The model under review builds one solid part; all positions refer to its coordinate system, in mm. A direction names the side the tool comes from. Coordinates: 2 decimals unless noted, no trailing zeros. Order: outer loops, then holes, each group sorted by start corner. A loop starts at its lowest first (then second) coordinate and runs counter-clockwise, first axis right, second up. Notation, with made-up numbers: (57, 57.25) -> (76, 57.25) arc R17 ccw to (76, 77.25) -> close; hole circle Ø5 at (19, -2.5). An arc over 180 degrees is marked (long way). Use one line per item in the form item = value. Start each with the question number.
(1) Take a section at C-C (y = 10.5). State the section outline as (x, z) points, then the cut area to 3 significant figures.
(2) For faces 1 (the flat face through (56, 0, 15)), 2 (the flat face through (35, 2, 2)), 3 (the flat face through (33.55, -2.5, 6.6)), 4 (the flat face through (36.45, -2.5, 6.6)), 5 (the flat face through (46, 0, 5)), list the 3-axis set-ups (+Z, -Z, +X, -X, +Y, -Y) from which the entire face can be reached by the end or side of a thin tool; tool diameter is ignored.
(3) Take a section at B-B (x = 57.5). State the section outline as (y, z) points, then the cut area to 3 significant figures.
(4) Take a section at D-D (x = 35). State the section outline as (y, z) points, then the cut area to 3 significant figures.
(5) Take a section at A-A (z = 12). State the section outline as (x, y) points.
(6) Wall thickness on line 1 along Z through (x, y) = (57.5, 10.7); line 2 along Z through (x, y) = (35, 3.5); line 3 along Z through (x, y) = (57.5, -1.5): over which ranges is each line inside the solid? List them lowest first.
(7) Mouldability with a two-part tool opening along X and no side actions: class faces 6 (the flat face through (33.55, -2.5, 17.3)), 7 (the cylindrical face through (36.6, 1.56, 11.93)), 8 (the flat face through (32, -2, 12)), 9 (the flat face through (36.45, -2.5, 17.3)) as +X half, -X half, draft (parallel to the pull), parting line (faces both ways), or undercut.
(8) Insertion check: pin 1 Ø12 at (x, y) = (56, 1.5) entering from +Z; pin 2 Ø0.5 at (y, z) = (-2.5, 19) entering from -X; pin 3 Ø1.5 at (y, z) = (-5.5, 16.5) entering from -X. Each pin has a flat end and moves straight along its axis. Give the tip position at first contact, or say it passes through.
```python
from build123d import *

# Parameters (mm, degrees)
MAIN_DEPTH                   = 22
ESQUISSE2_W                  = 10
ESQUISSE2_H                  = 8
ENL_V_MAT_EXTRU_1_DEPTH      = 19
ESQUISSE3_W                  = 21
ESQUISSE3_H                  = 10
ENL_V_MAT_EXTRU_2_DEPTH      = 10
ESQUISSE4_R                  = 3
ENL_V_MAT_EXTRU_3_DEPTH      = 1
ENL_V_MAT_EXTRU_3_DEPTH_BACK = 25
CONG_2_R                     = 5
ENL_V_START                  = -18
ESQUISSE6_W                  = 7
ESQUISSE6_H                  = 24
ENL_V_MAT_EXTRU_4_DEPTH      = 18
SKETCH1_W                    = 10
SKETCH1_H                    = 2
CUT_EXTRUDE1_DEPTH           = 19
SKETCH2_R                    = 1.6
CUT_EXTRUDE2_DEPTH           = 19
FILLET1_R                    = 1.5
CONG_3_R                     = 3
SKETCH3_W                    = 22
SKETCH3_H                    = 24
CUT_EXTRUDE3_DEPTH           = 39


with BuildPart() as part:
    # Esquisse1 → Main (new body)
    with BuildSketch(Plane.XY):
        Polygon((-12, -12), (12, -12), (12, -2), (15.55, -2), (15.55, -3), (18.45, -3), (18.45, -2), (22, -2), (22, 6), (12, 6), (12, 12), (-12, 12), align=None)
    extrude(amount=MAIN_DEPTH)

    # Esquisse2 → Enlèv. mat.-Extru.1 (cut, through all)
    with BuildSketch(Plane(origin=(6, 0, 0), x_dir=(0, 0, -1), z_dir=(1, 0, 0))):
        with Locations((-5, 2)):
            Rectangle(ESQUISSE2_W, ESQUISSE2_H)
    extrude(amount=-ENL_V_MAT_EXTRU_1_DEPTH, mode=Mode.SUBTRACT)

    # Esquisse3 → Enlèv. mat.-Extru.2 (cut)
    with BuildSketch(Plane(origin=(0, 0, 0), x_dir=(-1, 0, 0), z_dir=(0, 0, -1))):
        with Locations((1.5, -7)):
            Rectangle(ESQUISSE3_W, ESQUISSE3_H)
    extrude(amount=-ENL_V_MAT_EXTRU_2_DEPTH, mode=Mode.SUBTRACT)

    # Esquisse4 → Enlèv. mat.-Extru.3 (cut, two sides)
    with BuildSketch(Plane(origin=(0, 12, 0), x_dir=(1, 0, 0), z_dir=(0, 1, 0))) as enl_v_mat_extru_3_sk:
        with Locations((-5.5, -5)):
            Circle(ESQUISSE4_R)
    extrude(amount=ENL_V_MAT_EXTRU_3_DEPTH, mode=Mode.SUBTRACT)
    extrude(enl_v_mat_extru_3_sk.sketch, amount=-ENL_V_MAT_EXTRU_3_DEPTH_BACK, mode=Mode.SUBTRACT)

    # Congé2
    cong_2_edges = [part.edges().sort_by_distance(p)[0] for p in [
        (-12, 9, 0),
        (6, 6, 5),
    ]]
    fillet(cong_2_edges, radius=CONG_2_R)

    # Esquisse6 → Enlèv. mat.-Extru.4 (cut)
    with BuildSketch(Plane.ZY.offset(12).offset(ENL_V_START)):
        with Locations((18.5, 0)):
            Rectangle(ESQUISSE6_W, ESQUISSE6_H)
    extrude(amount=ENL_V_MAT_EXTRU_4_DEPTH, mode=Mode.SUBTRACT)

    # Sketch1 → Cut-Extrude1 (cut, through all)
    with BuildSketch(Plane(origin=(0, 6, 0), x_dir=(1, 0, 0), z_dir=(0, 1, 0))):
        with Locations((17, -1)):
            Rectangle(SKETCH1_W, SKETCH1_H)
    extrude(amount=-CUT_EXTRUDE1_DEPTH, mode=Mode.SUBTRACT)

    # Sketch2 → Cut-Extrude2 (cut, through all)
    with BuildSketch(Plane(origin=(0, 6, 0), x_dir=(1, 0, 0), z_dir=(0, 1, 0))):
        with Locations((17, -12)):
            Circle(SKETCH2_R)
    extrude(amount=-CUT_EXTRUDE2_DEPTH, mode=Mode.SUBTRACT)

    # Fillet1
    fillet1_edges = [part.edges().sort_by_distance(p)[0] for p in [
        (12, 6, 12),
    ]]
    fillet(fillet1_edges, radius=FILLET1_R)

    # Congé3
    cong_3_edges = [part.edges().sort_by_distance(p)[0] for p in [
        (6, 0, 15),
    ]]
    fillet(cong_3_edges, radius=CONG_3_R)


with BuildPart() as body_2:
    # Mirror1: mirrored copy
    add(part.part.mirror(Plane(origin=(26, 0, 0), x_dir=(0, 0, 1), z_dir=(1, 0, 0))))


with BuildPart() as part_1:
    add(part.part)

    # Sketch3 → Cut-Extrude3 (cut, through all)
    with BuildSketch(Plane(origin=(26, 0, 0), x_dir=(0, 0, -1), z_dir=(1, 0, 0))):
        with Locations((-11, 0)):
            Rectangle(SKETCH3_W, SKETCH3_H)
    extrude(amount=-CUT_EXTRUDE3_DEPTH, mode=Mode.SUBTRACT)


solid = body_2.part
```
Findings:
q1.outline = (40, 0) -> (59, 0) arc R5 ccw to (64, 5) -> (64, 15) -> (49, 15) arc R3 cw to (46, 18) -> (46, 22) -> (40, 22) -> close; hole circle Ø6 at (57.5, 5)
q1.area = 370 mm²
q2.face_1 = +Z, +X, +Y, -Y
q2.face_2 = -Z, -X, +Y, -Y
q2.face_3 = +Z, -Z, -X, -Y
q2.face_4 = +Z, -Z, -Y
q2.face_5 = -Z, +X, -Y
q3.outline = (-12, 10) -> (6, 10) -> (6, 8) -> (12, 8) -> (12, 15) -> (-12, 15) -> close; (6, 0) -> (12, 0) -> (12, 2) -> (6, 2) -> close
q3.area = 144 mm²
q4.outline = (-3, 2) -> (6, 2) -> (6, 10.4) -> (-3, 10.4) -> close; (-3, 13.6) -> (6, 13.6) -> (6, 22) -> (-3, 22) -> close
q4.area = 151 mm²
q5.outline = (30, -2) -> (33.4, -2) -> (33.4, 6) -> (30, 6) -> close; (36.6, -2) -> (40, -2) -> (40, -12) -> (64, -12) -> (64, 12) -> (40, 12) -> (40, 7.5) arc R1.5 cw to (38.5, 6) -> (36.6, 6) -> close
q6.line_1 = 0 to 2, 8 to 15
q6.line_2 = 2 to 10.4, 13.6 to 22
q6.line_3 = 10 to 15
q7.face_6 = -X half
q7.face_7 = undercut
q7.face_8 = draft
q7.face_9 = undercut
q8.pin_1 = 15
q8.pin_2 = 33.55
q8.pin_3 = 40
